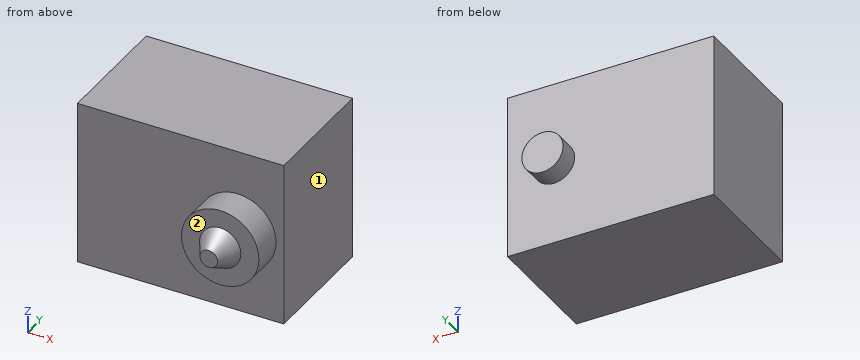
from build123d import *

# Parameters (mm, degrees)
SKETCH_1_W      = 20
SKETCH_1_H      = 16
EXTRUDE_1_DEPTH = 12
SKETCH_2_R      = 2
EXTRUDE_2_DEPTH = 2
SKETCH_3_R      = 3.75
EXTRUDE_3_DEPTH = 3
SKETCH_4_R      = 2
EXTRUDE_4_DEPTH = 2
EXTRUDE_4_TAPER = 30


with BuildPart() as part:
    # Эскиз1 → Бобышка-Вытянуть1 (new body)
    with BuildSketch(Plane(origin=(0, 0, 0), x_dir=(1, 0, 0), z_dir=(0, 1, 0))):
        with Locations((10, 8)):
            Rectangle(SKETCH_1_W, SKETCH_1_H)
    extrude(amount=EXTRUDE_1_DEPTH)

    # Эскиз2 → Бобышка-Вытянуть2 (add)
    with BuildSketch(Plane(origin=(0, 12, 0), x_dir=(1, 0, 0), z_dir=(0, 1, 0))):
        with Locations(Location((15.5, 8, 0), (0, 0, 90))):
            Circle(SKETCH_2_R)
    extrude(amount=EXTRUDE_2_DEPTH)

    # Эскиз3 → Бобышка-Вытянуть3 (add)
    with BuildSketch(Plane.XZ):
        with Locations(Location((15.5, -8, 0), (0, 0, 270))):
            Circle(SKETCH_3_R)
    extrude(amount=EXTRUDE_3_DEPTH)

    # Эскиз4 → Бобышка-Вытянуть4 (add)
    with BuildSketch(Plane.XZ.offset(3)):
        with Locations(Location((15.5, -8, 0), (0, 0, 270))):
            Circle(SKETCH_4_R)
    extrude(amount=EXTRUDE_4_DEPTH, taper=EXTRUDE_4_TAPER)


solid = part.part
The listing builds one solid part. Answer for the finished solid, in the listing's coordinates (mm). Face numbers are marked on the shaded views. A direction names the side the tool comes from. Coordinates: 2 decimals unless noted, no trailing zeros. Order: outer loops, then holes, each group sorted by start corner. A loop starts at its lowest first (then second) coordinate and runs counter-clockwise, first axis right, second up.
Q1. Given P1, Ø3, axis at x = 16, z = -4.5, coming from the +Y side; P2, Ø8, axis at x = 8, z = -9.5, coming from the -Y side, each flat-ended and moving along its own axis, determine where each tip first touches the part or whether it passes through.
Q2. A cutting plane is placed at B-B, the plane x = 3. Write down the section's boundary in (y, z), and give its area (3 significant figures).
Q3. A cutting plane is placed at C-C, the plane z = -10.5. Write down the section's boundary in (x, y), and give its area (3 significant figures).
Q4. A cutting plane is placed at A-A, the plane z = -8. Write down the section's boundary in (x, y).
Q5. Consider line 1 (Y direction, x = 9.5, z = -5); line 2 (Z direction, x = 15.5, y = 12.5); line 3 (X direction, y = 12.75, z = -6.75). Determine where each line is inside the solid, lowest interval first.
Q6. Which of the six approach directions +Z, -Z, +X, -X, +Y, -Y give full straight-line access (tool end or side, diameter ignored) to the marked faces 1 and 2?
Answers follow:
1. P1: stops at y = 12
1. P2: stops at y = -3
2. outline: (0, -16) - (12, -16) - (12, 0) - (0, 0) - close
2. area: 192 mm2
3. outline: (0, 0) - (12.7, 0) - (12.7, -3) - (18.3, -3) - (18.3, 0) - (20, 0) - (20, 12) - (0, 12) - close
3. area: 257 mm2
4. outline: (0, 0) - (11.75, 0) - (11.75, -3) - (13.5, -3) - (14.65, -5) - (16.35, -5) - (17.5, -3) - (19.25, -3) - (19.25, 0) - (20, 0) - (20, 12) - (17.5, 12) - (17.5, 14) - (13.5, 14) - (13.5, 12) - (0, 12) - close
5. line 1: y = 0 to 12
5. line 2: z = -10 to -6
5. line 3: x = 13.94 to 17.06
6. face 1: +Z, -Z, +X, +Y, -Y
6. face 2: -Y
